from build123d import *

# Parameters (mm, degrees)
STRUCTURAL_MEMBER1_DEPTH       = 770
F_10_0_10_DIAMETER_HOLE1_D     = 10
F_10_0_10_DIAMETER_HOLE1_DEPTH = 11
F_10_0_10_DIAMETER_HOLE1_TIP   = 3.004303095
SKETCH28_R                     = 5
CUT_EXTRUDE1_DEPTH             = 773.026553947
F_10_0_10_DIAMETER_HOLE2_D     = 10
F_10_0_10_DIAMETER_HOLE2_DEPTH = 11
F_10_0_10_DIAMETER_HOLE2_TIP   = 3.004303095
F_5_0_5_DIAMETER_HOLE1_D       = 5
F_5_0_5_DIAMETER_HOLE1_DEPTH   = 11
F_5_0_5_DIAMETER_HOLE1_TIP     = 1.502151548
SKETCH33_R                     = 2.5
CUT_EXTRUDE2_DEPTH             = 10


with BuildPart() as part:
    # Sketch11 → Structural Member1 (new body)
    with BuildSketch(Plane(origin=(0, 0, 0), x_dir=(-1, 0, 0), z_dir=(0, 0, -1))):
        with BuildLine():
            Line((25, 50), (0, 50))
            Line((0, 50), (0, 0))
            Line((0, 0), (25, 0))
            Line((25, 0), (25, 2))
            ThreePointArc((25, 2), (24.414213562, 3.414213562), (23, 4))
            Line((23, 4), (9, 4))
            ThreePointArc((9, 4), (6.171572875, 5.171572875), (5, 8))
            Line((5, 8), (5, 42))
            ThreePointArc((5, 42), (6.171572875, 44.828427125), (9, 46))
            Line((9, 46), (23, 46))
            ThreePointArc((23, 46), (24.414213562, 46.585786438), (25, 48))
            Line((25, 48), (25, 50))
        make_face()
    extrude(amount=STRUCTURAL_MEMBER1_DEPTH)

    # Ø10.0 (10) Diameter Hole1
    with Locations(Plane(origin=(0, 0, 0), x_dir=(0, 0, -1), z_dir=(1, 0, 0))):
        with Locations((550, 25), (640, 25)):
            Hole(F_10_0_10_DIAMETER_HOLE1_D / 2, depth=F_10_0_10_DIAMETER_HOLE1_DEPTH)
            with Locations((0, 0, -(F_10_0_10_DIAMETER_HOLE1_DEPTH + F_10_0_10_DIAMETER_HOLE1_TIP / 2))):  # 118° drill point
                Cone(0, F_10_0_10_DIAMETER_HOLE1_D / 2, F_10_0_10_DIAMETER_HOLE1_TIP, mode=Mode.SUBTRACT)

    # Sketch28 → Cut-Extrude1 (cut, through all)
    with BuildSketch(Plane.XZ):
        with Locations((-16, -295)):
            Circle(SKETCH28_R)
    extrude(amount=-CUT_EXTRUDE1_DEPTH, mode=Mode.SUBTRACT)

    # Ø10.0 (10) Diameter Hole2
    with Locations(Plane(origin=(0, 0, 0), x_dir=(0, 0, -1), z_dir=(1, 0, 0))):
        with Locations((43.5, 25), (246.5, 25)):
            Hole(F_10_0_10_DIAMETER_HOLE2_D / 2, depth=F_10_0_10_DIAMETER_HOLE2_DEPTH)
            with Locations((0, 0, -(F_10_0_10_DIAMETER_HOLE2_DEPTH + F_10_0_10_DIAMETER_HOLE2_TIP / 2))):  # 118° drill point
                Cone(0, F_10_0_10_DIAMETER_HOLE2_D / 2, F_10_0_10_DIAMETER_HOLE2_TIP, mode=Mode.SUBTRACT)

    # Ø5.0 (5) Diameter Hole1
    with Locations(Plane(origin=(0, 0, 0), x_dir=(0, 0, -1), z_dir=(1, 0, 0))):
        with Locations((515, 33.95), (675, 33.95), (495, 33.95), (695, 33.95)):
            Hole(F_5_0_5_DIAMETER_HOLE1_D / 2, depth=F_5_0_5_DIAMETER_HOLE1_DEPTH)
            with Locations((0, 0, -(F_5_0_5_DIAMETER_HOLE1_DEPTH + F_5_0_5_DIAMETER_HOLE1_TIP / 2))):  # 118° drill point
                Cone(0, F_5_0_5_DIAMETER_HOLE1_D / 2, F_5_0_5_DIAMETER_HOLE1_TIP, mode=Mode.SUBTRACT)

    # Sketch33 → Cut-Extrude2 (cut)
    with BuildSketch(Plane(origin=(0, 0, 0), x_dir=(0, 0, -1), z_dir=(1, 0, 0))):
        with Locations(Location((505.309927761, 22.5, 0), (0, 0, 90))):
            Circle(SKETCH33_R)
        with Locations(Location((325.309927761, 22.5, 0), (0, 0, 90))):
            Circle(SKETCH33_R)
    extrude(amount=-CUT_EXTRUDE2_DEPTH, mode=Mode.SUBTRACT)


solid = part.part
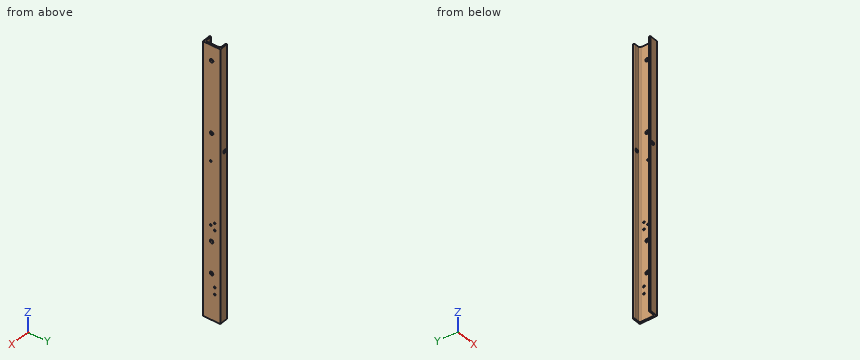
Read the model definition and answer for the solid it produces. Units are mm, in the model's axes. Round coordinates to 2 decimals unless told otherwise and drop trailing zeros. Loops run counter-clockwise (first coordinate to the right, second up) from the corner with the lowest first, then second, coordinate; pieces in that order, holes last.
Q1. Section B-B on z = -276.5 is taken. Write down the section's boundary in (x, y).
Q2. Section A-A on x = -16 is taken. Write down the section's boundary in (y, z).
Q3. Consider probe 1 along Y at (x, z) = (-1.35, -495); probe 2 along Y at (x, z) = (-15, -376.5); probe 3 along X at (y, z) = (16.5, -198). Determine where each line is inside the solid, lowest interval first.
Q4. Each of these flat-tipped pins is pushed along its axis until it touches: pin 1 (5 mm diameter, centred on y = 43, z = -470, fed in from -X); pin 2 (16 mm diameter, centred on y = 25, z = -246.5, fed in from -X); pin 3 (6 mm diameter, centred on x = -11.5, y = 41, fed in from -Z). Where does it stop, or does it pass through?
Output:
1. outline: (-25, 0) - (0, 0) - (0, 50) - (-25, 50) - (-25, 48) arc R2 ccw to (-23, 46) - (-9, 46) arc R4 cw to (-5, 42) - (-5, 8) arc R4 cw to (-9, 4) - (-23, 4) arc R2 ccw to (-25, 2) - close
2. outline: (0, -770) - (4, -770) - (4, -300) - (0, -300) - close; (0, -290) - (4, -290) - (4, 0) - (0, 0) - close; (46, -770) - (50, -770) - (50, -300) - (46, -300) - close; (46, -290) - (50, -290) - (50, 0) - (46, 0) - close
3. probe 1: y = 0 to 31.45, 36.45 to 50
3. probe 2: y = 0 to 4, 46 to 50
3. probe 3: x = -5 to 0
4. pin 1: stops at x = -7.06
4. pin 2: stops at x = -5
4. pin 3: passes through
